Model file for the job. Use its own axes, mm. A direction names the side the tool comes from. Coordinates: 2 decimals unless noted, no trailing zeros. Order: outer loops, then holes, each group sorted by start corner. A loop starts at its lowest first (then second) coordinate and runs counter-clockwise, first axis right, second up.
Autodesk Inventor part; units mm, degrees
ref_plane "YZ Plane" through (0, 0, 0) normal (1, 0, 0) x (0, 1, 0)
ref_plane "XZ Plane" through (0, 0, 0) normal (0, 1, 0) x (-1, 0, 0)
ref_plane "XY Plane" through (0, 0, 0) normal (0, 0, 1) x (1, 0, 0)
sketch "Sketch1" plane through (0, 0, 0) normal (0, 0, 1) x (1, 0, 0)
  line L0 (0, 0) -> (22, 0)
  line L1 (22, 0) -> (22, 12)
  line L2 (22, 12) -> (0, 12)
  line L3 (0, 12) -> (0, 0)
  dimension "d0" = 22
  dimension "d1" = 12
extrude "Extrusion1" add sketch "Sketch1" along normal blind 1.5
sketch "Sketch2" plane through (0, 0, 1.5) normal (0, 0, 1) x (1, 0, 0)
  line L0 (22, 0) -> (22, 12)
  line L1 (0, 12) -> (0, 0)
  line L2 (22, 8) -> (0, 8)
  line L3 (0, 8) -> (0, 2)
  line L4 (0, 2) -> (22, 2)
  line L5 (22, 2) -> (22, 8)
  line L6 (0, 0) -> (22, 0)
  point P0 (0, 8)
  dimension "d4" = 2
  dimension "d5" = 6
extrude "Extrusion2" add sketch "Sketch2" along normal blind 9.5 contours L4 L1 L2 L0
sketch "Sketch3" plane through (0, 8, 1.5) normal (0, 1, 0) x (1, 0, 0)
  line L0 (0, -9.5) -> (22, -9.5)
  circle A0 centre (9, -9.5) radius 8
  line L1 (0, 0) -> (0, -9.5)
  point P0 (0, 1.5)
  point P1 (17, -9.5)
  point P2 (1, -9.5)
  dimension "d8" = 16
  dimension "d9" = 1
extrude "Extrusion3" cut sketch "Sketch3" against normal through all contours A0 L0 picked at (10.996, -7.7317)
sketch "Sketch4" plane through (0, 0, 1.5) normal (0, 0, 1) x (1, 0, 0)
  line L0 (0, 0) -> (22, 0)
  line L1 (22, 2) -> (0, 2)
  line L2 (0, 0) -> (22, 0)
  line L3 (22, 0) -> (22, 2)
  line L4 (22, 2) -> (0, 2)
  line L5 (0, 2) -> (0, 0)
  line L6 (22, 0) -> (22, 12)
  line L7 (0, 12) -> (0, 0)
  line L8 (22, 8) -> (0, 8)
  line L9 (0, 8) -> (0, 10)
  line L10 (0, 10) -> (22, 10)
  line L11 (22, 10) -> (22, 8)
extrude "Extrusion4" add sketch "Sketch4" along normal up to surface (9.5 mm away) contours L5 L1 L3 L0 | L7 L10 L6 L8
sketch "Sketch5" plane through (0, 0, 0) normal (0, -1, 0) x (1, 0, 0)
  arc A0 (1, 11) -> (17, 11) centre (9, 11) ccw
  circle A1 centre (9, 11) radius 6
  point P0 (0, 0)
extrude "Extrusion5" cut sketch "Sketch5" against normal through all
sketch "Sketch6" plane through (0, 0, 11) normal (0, 0, 1) x (1, 0, 0)
  circle A0 centre (19.5, 5) radius 1.25
  line L0 (22, 10) -> (22, 0)
  line L1 (22, 0) -> (15, 0)
  point P0 (0, 0)
  dimension "d16" = 2.5
  dimension "d17" = 2.5
  dimension "d18" = 5
extrude "Extrusion6" cut sketch "Sketch6" against normal through all
thicken "Thicken1" operation add thickness 0.5 both sides no extend neighbours yes toward (1, 0, 0) faces at (0, 3.3333, 4.1667) (14.6667, 12, 1) (22, 3.3333, 4.1667)
chamfer "Chamfer1" distance 1.5 angle 45 1 edges at (18.25, 5, 0)
properties part number "bearingholder"
Q1. Which spindle directions (+Z, -Z, +X, -X, +Y, -Y) get a long thin tool onto all of the face, cutting with end or side? Do faces 5 (the face through (0.5, 6, 5)), 6 (the face through (11, 11, 1.5)), 7 (the face through (9, 8, 4)). Say none if no direction does.
Established:
face 5: +Z, -Z, -X, +Y, -Y
face 6: +Z, +X, -X, +Y
face 7: +Z
Q2. Probe line 1 (Y direction, x = 19.5, z = 4.5); line 2 (Y direction, x = 9.25, z = 3.25); line 3 (X direction, y = 5.75, z = 8.5). List the from-to ranges inside material, lowest first.
Established:
line 1: y = 0 to 3.75, 6.25 to 10
line 2: y = 0 to 2, 8 to 10
line 3: x = 0.5 to 1.4, 16.6 to 18.5, 20.5 to 21.5
Q3. Cut at B-B, the plane z = 10. List the corners of the cut face in (x, y), plus the area to 3 significant figures.
Established:
outline: (0.5, 0) - (3.08, 0) - (3.08, 2) - (1.06, 2) - (1.06, 8) - (3.08, 8) - (3.08, 10) - (0.5, 10) - close; (14.92, 0) - (21.5, 0) - (21.5, 10) - (14.92, 10) - (14.92, 8) - (16.94, 8) - (16.94, 2) - (14.92, 2) - close; hole circle Ø2.5 at (19.5, 5)
area: 62.5 mm2
Q4. Cut at C-C, the plane x = 19.5. List the corners of the cut face in (y, z), plus the area to 3 significant figures.
Established:
outline: (0, 0) - (2.25, 0) - (3.75, 1.5) - (3.75, 11) - (0, 11) - close; (6.25, 1.5) - (7.75, 0) - (11.5, 0) - (11.5, 1.5) - (10, 1.5) - (10, 11) - (6.25, 11) - close
area: 82.5 mm2
Q5. Cut at A-A, the plane y = 5. List the corners of the cut face in (x, z), plus the area to 3 significant figures.
Established:
outline: (0.5, 0) - (16.75, 0) - (18.25, 1.5) - (18.25, 11) - (17, 11) arc R8 cw to (1, 11) - (0.5, 11) - close; (20.75, 1.5) - (21.5, 0.75) - (21.5, 11) - (20.75, 11) - close
area: 101 mm2
Q6. Mould opens along Y. For faces 1 (the face through (11, 11.5, 1)), 2 (the face through (9, 9, 5)), 3 (the face through (9, 5, 3)), 4 (the face through (11, 0, 4)) say: pulls with the +Y half, pulls with the -Y half, needs draft (parallel to the pull), parting line crosses it, or undercut.
Established:
face 1: pulls with the +Y half
face 2: needs draft
face 3: undercut
face 4: pulls with the -Y half
Q7. Cut at D-D, the plane x = 9. List the corners of the cut face in (y, z), plus the area to 4 significant figures.
Established:
outline: (0, 0) - (11.5, 0) - (11.5, 1.5) - (10, 1.5) - (10, 5) - (8, 5) - (8, 3) - (2, 3) - (2, 5) - (0, 5) - close
area: 40.25 mm2
Q8. Drop flat-ended pins along their axis: P1, Ø1.5, axis at x = 18.5, y = 6.5, coming from the -Z side; P2, Ø6.5, axis at x = 7, z = 7, coming from the +Y side. Give the stop position or say it passes through.
Established:
P1: stops at z = 0.2
P2: stops at y = 10
